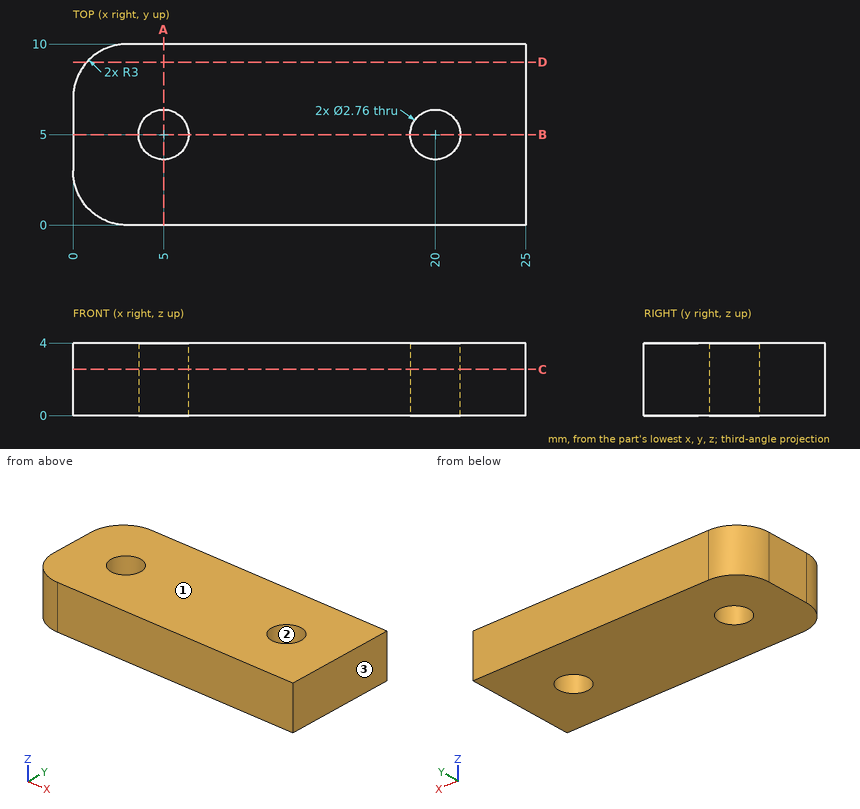
Input: dimensioned drawing with shaded views. Units: mm. Origin: part minimum x, y, z. Coordinates: 2 decimals unless noted, no trailing zeros. Order: outer loops, then holes, each group sorted by start corner. A loop starts at its lowest first (then second) coordinate and runs counter-clockwise, first axis right, second up. Notation, with made-up numbers: (64, 7.25) - (121, 7.25) arc R19 cw to (121, 13.25) - close; hole circle Ø5 at (73, 68). An arc over 180 degrees is marked (long way). Return JSON: item names as keys, results as strings. Group by question number.
1. Pin query (flat end, axial travel): pin 1 (1 mm diameter, centred on x = 5.5, y = 4.5, fed in from +Z). Return the tip coordinate at first contact, or that it passes through.
2. Material intervals for line 1 along X through (y, z) = (5, 1.65); line 2 along Y through (x, z) = (5, 1.45); line 3 along X through (y, z) = (6, 2.9), sorted ascending. Write a range as [from, to].
3. Cut plane D-D (y = 9). Output: boundary loops of the cut face in (x, z).
4. Cut plane C-C (z = 2.55). Output: boundary loops of the cut face in (x, y), plus the area to 3 significant figures.
5. Pull-direction query (X, two-part tool) for the marked faces 1, 2 and 3; classes: pulls with the +X half, pulls with the -X half, needs draft (parallel to the pull), parting line crosses it, or undercut.
6. Cut plane B-B (y = 5). Output: boundary loops of the cut face in (x, z), plus the area to 3 significant figures.
7. Cut plane A-A (x = 5). Output: boundary loops of the cut face in (y, z), plus the area to 3 significant figures.
Resolved:
{
 "1": {"pin 1": "passes through"},
 "2": {"line 1": "x = [0, 3.62], [6.38, 18.62], [21.38, 25]", "line 2": "y = [0, 3.62], [6.38, 10]", "line 3": "x = [0, 4.05], [5.95, 19.05], [20.95, 25]"},
 "3": {"outline": "(0.76, 0) - (25, 0) - (25, 4) - (0.76, 4) - close"},
 "4": {"outline": "(0, 3) arc R3 ccw to (3, 0) - (25, 0) - (25, 10) - (3, 10) arc R3 ccw to (0, 7) - close; hole circle Ø2.76 at (5, 5); hole circle Ø2.76 at (20, 5)", "area": "234 mm²"},
 "5": {"face 1": "needs draft", "face 2": "undercut", "face 3": "pulls with the +X half"},
 "6": {"outline": "(0, 0) - (3.62, 0) - (3.62, 4) - (0, 4) - close; (6.38, 0) - (18.62, 0) - (18.62, 4) - (6.38, 4) - close; (21.38, 0) - (25, 0) - (25, 4) - (21.38, 4) - close", "area": "77.9 mm²"},
 "7": {"outline": "(0, 0) - (3.62, 0) - (3.62, 4) - (0, 4) - close; (6.38, 0) - (10, 0) - (10, 4) - (6.38, 4) - close", "area": "29.0 mm²"}
}
